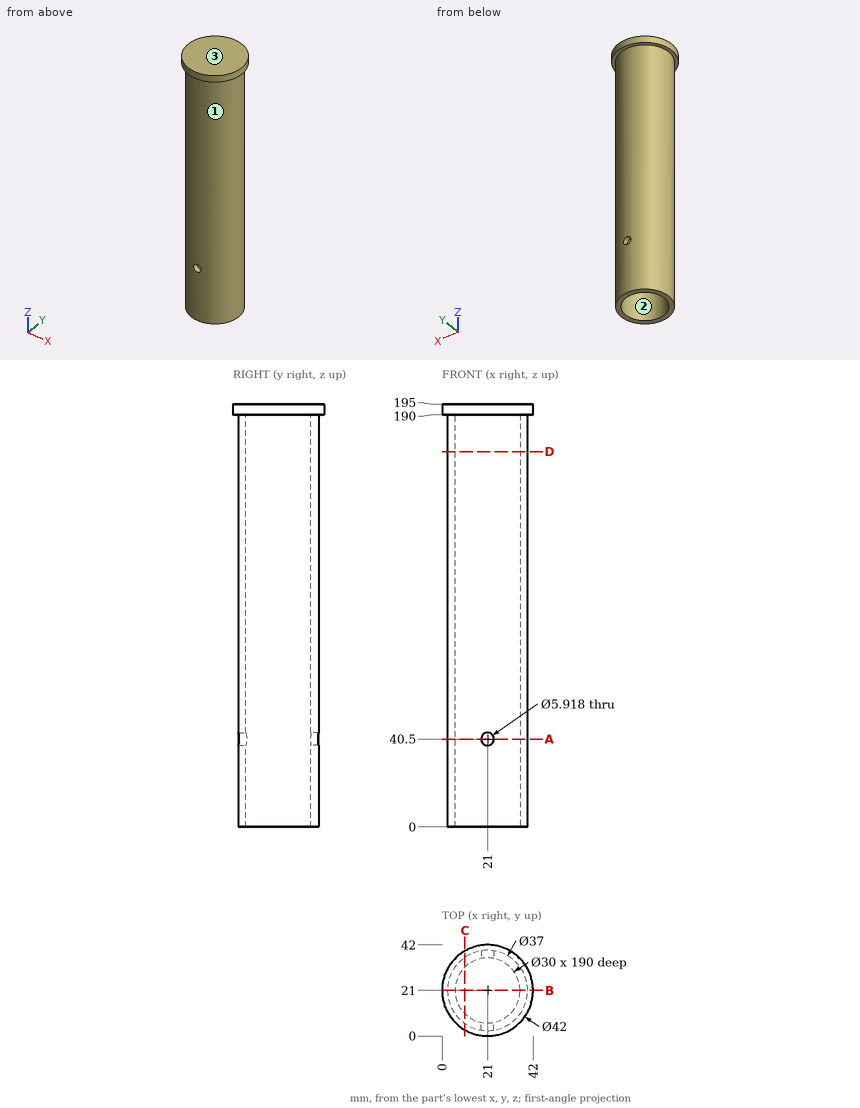
Could you check a few things on this drawing? It's one solid part, dimensions in mm from its lowest x, y, z. Coordinates: 2 decimals unless noted, no trailing zeros. Write each loop counter-clockwise with the first axis right and the second up, starting at its lowest first coordinate (ties: lowest second). Pieces come first, ordered by that corner, then holes. Notation, with made-up numbers: (40.5, 65.5) - (92.5, 65.5) arc R18 cw to (92.5, 88.5) - close; hole circle Ø10 at (33.5, 5.25). An arc over 180 degrees is marked (long way). Use one line per item in the form item = value.
1) I'm going to push flat-ended pins straight in: P1, Ø1.5, axis at y = 9.5, z = 90, coming from the +X side (1 decimal); P2, Ø12, axis at y = 35, z = 130, coming from the +X side; P3, Ø1, axis at x = 18, z = 84.5, coming from the +Y side. Where does each tip first touch, or does it pass through?
Solved:
P1 = 36.1
P2 = 37.68
P3 = 39.33
2) Suppose I cut it at B-B, the plane y = 21. Write out the boundary of the cut face in (x, z).
Solved:
outline = (0, 190) - (2.5, 190) - (2.5, 0) - (6, 0) - (6, 190) - (36, 190) - (36, 0) - (39.5, 0) - (39.5, 190) - (42, 190) - (42, 195) - (0, 195) - close
3) Suppose I cut it at C-C, the plane x = 10.5. Write out the boundary of the cut face in (y, z).
Solved:
outline = (2.81, 190) - (5.77, 190) - (5.77, 0) - (10.29, 0) - (10.29, 190) - (31.71, 190) - (31.71, 0) - (36.23, 0) - (36.23, 190) - (39.19, 190) - (39.19, 195) - (2.81, 195) - close
4) Suppose I cut it at A-A, the plane z = 40.5. Write out the boundary of the cut face in (x, y) (1 decimal), plus the area to 3 significant figures.
Solved:
outline = (18, 2.7) - (18, 6.3) arc R15 cw to (18, 35.7) - (18, 39.3) arc R18.5 ccw to start; (24, 2.7) arc R18.5 ccw to (24, 39.3) - (24, 35.7) arc R15 cw to (24, 6.3) - close
area = 327 mm2
5) Suppose I cut it at D-D, the plane z = 173. Write out the boundary of the cut face in (x, y).
Solved:
outline = circle Ø37 at (21, 21); hole circle Ø30 at (21, 21)
6) Thinking about a two-plate mould opening in Y: for the marked faces 1, 2 and 3, which applies, released by +Y, released by -Y, zero draft, split by the parting line, or undercut?
Solved:
face_1 = split by the parting line
face_2 = undercut
face_3 = zero draft
7) I need wall thicknesses on line 1 (Z direction, x = 21, y = 4); line 2 (Z direction, x = 10, y = 24); line 3 (Y direction, x = 21, z = 83). Which ranges of each line are inside material? Lowest first, please.
Solved:
line_1 = 0 to 37.54, 43.46 to 195
line_2 = 190 to 195
line_3 = 2.5 to 6, 36 to 39.5
